Here's how the part is built. I have some questions about the finished solid (model axes, mm). A direction names the side the tool comes from. Coordinates: 2 decimals unless noted, no trailing zeros. Write each loop counter-clockwise with the first axis right and the second up, starting at its lowest first coordinate (ties: lowest second). Pieces come first, ordered by that corner, then holes. Notation, with made-up numbers: (-33.5, 71.5) - (10.5, 71.5) arc R15 ccw to (10.5, 87.5) - close; hole circle Ø2 at (54, 3.25). An arc over 180 degrees is marked (long way). Answer in a Markdown table with one row per item. Add a question column.
Item 1: Imagine slicing it at C-C (y = 3.15). Please give me the cut outline in (x, z).
Item 2: Which directions (+Z, -Z, +X, -X, +Y, -Y) give clear straight access to the entire face, cutting with the end or side of a thin tool? Please do faces 1 (the face through (2, 3, -3)), 2 (the face through (3, 2, 0)), 3 (the face through (1, 1, -2)).
Item 3: Imagine slicing it at B-B (z = -0.8). Please give me the cut outline in (x, y), plus the area to 3 significant figures.
Item 4: If I drill on probe 1 along Y at (x, z) = (1.2, -2); probe 2 along X at (y, z) = (1.9, -2.55); probe 3 along X at (y, z) = (4.05, -1.35), over which ranges is the centre line in solid material (lowest first)? Write a range as from..to.
Item 5: Imagine slicing it at D-D (y = 0.45). Please give me the cut outline in (x, z).
Item 6: Imagine slicing it at A-A (x = 2.9). Please give me the cut outline in (y, z).
from build123d import *

# Parameters (mm, degrees)
SKETCH2_W           = 6
SKETCH2_H           = 4
BOSS_EXTRUDE1_DEPTH = 5
SKETCH3_W           = 1
SKETCH3_H           = 3
CUT_EXTRUDE1_DEPTH  = 5
CUT_EXTRUDE3_DEPTH  = 2


with BuildPart() as part:
    # Sketch2 → Boss-Extrude1 (new body)
    with BuildSketch(Plane(origin=(0, 0, 0), x_dir=(1, 0, 0), z_dir=(0, 1, 0))):
        with Locations((3, 2)):
            Rectangle(SKETCH2_W, SKETCH2_H)
    extrude(amount=BOSS_EXTRUDE1_DEPTH)

    # Sketch3 → Cut-Extrude1 (cut)
    with BuildSketch(Plane.XY):
        with Locations((0.5, 1.5)):
            Rectangle(SKETCH3_W, SKETCH3_H)
    extrude(amount=-CUT_EXTRUDE1_DEPTH, mode=Mode.SUBTRACT)

    # Sketch5 → Cut-Extrude3 (cut)
    with BuildSketch(Plane(origin=(0, 5, 0), x_dir=(1, 0, 0), z_dir=(0, 1, 0))):
        Polygon((0, 0), (4, 4), (0, 4), align=None)
    extrude(amount=-CUT_EXTRUDE3_DEPTH, mode=Mode.SUBTRACT)


solid = part.part
Here are the results:
| question | item | result |
|---|---|---|
| 1 | outline | (0, 0) - (4, -4) - (6, -4) - (6, 0) - close |
| 2 | face 1 | -Z, -X, +Y |
| 2 | face 2 | +Z, +X, -X, +Y, -Y |
| 2 | face 3 | +Z, -Z, -X, -Y |
| 3 | outline | (0.8, 3) - (1, 3) - (1, 0) - (6, 0) - (6, 5) - (0.8, 5) - close |
| 3 | area | 25.4 mm2 |
| 4 | probe 1 | y = 0..3 |
| 4 | probe 2 | x = 1..6 |
| 4 | probe 3 | x = 1.35..6 |
| 5 | outline | (1, -4) - (6, -4) - (6, 0) - (1, 0) - close |
| 6 | outline | (0, -4) - (3, -4) - (3, -2.9) - (5, -2.9) - (5, 0) - (0, 0) - close |
